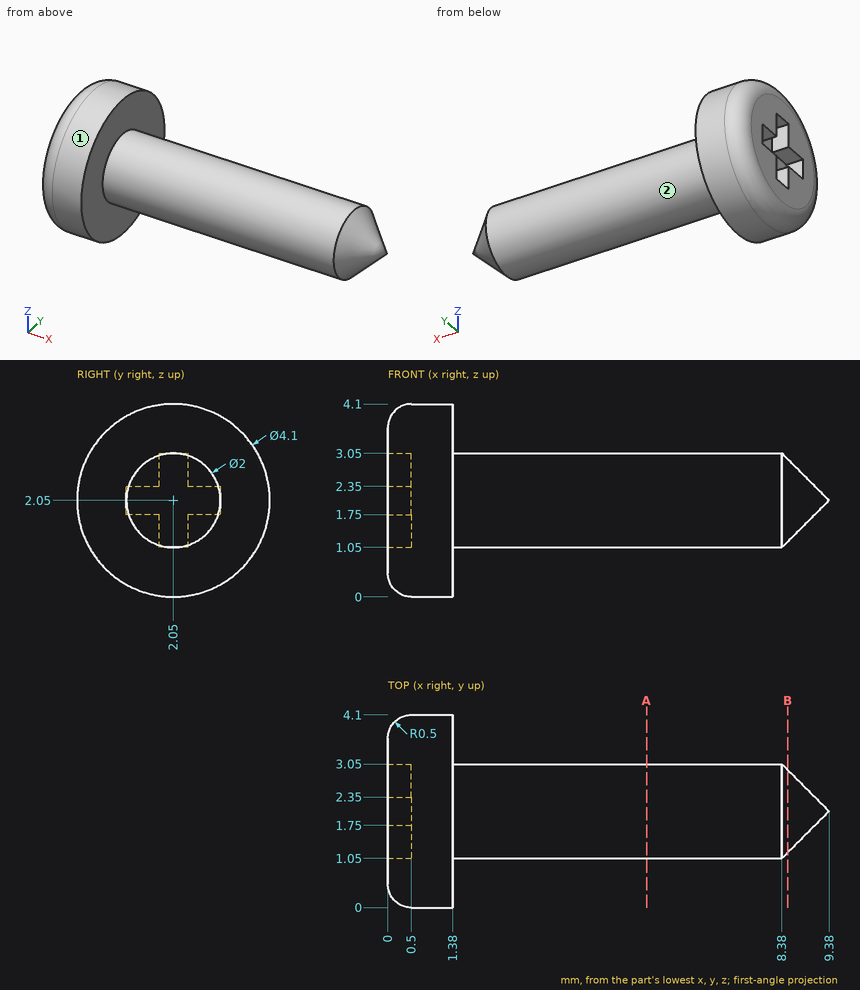
Input: dimensioned drawing with shaded views. Units: mm. Origin: part minimum x, y, z. A direction names the side the tool comes from. Give positions to 0.01 mm unless a question says otherwise; leave off trailing zeros. Write each loop counter-clockwise with the first axis right and the second up, starting at its lowest first coordinate (ties: lowest second). Pieces come first, ordered by that corner, then holes. Notation, with made-up numbers: (0.5, 41.5) - (12.5, 41.5) arc R22 cw to (12.5, 52.5) - close; hole circle Ø11 at (-38.5, 33.25). An arc over 180 degrees is marked (long way). One line per item, written item: value. Start each with the question number.
Q1. Material intervals for probe 1 along X at (y, z) = (1.4, 0.75); probe 2 along Y at (x, z) = (3, 1.2); probe 3 along Z at (x, y) = (3, 1.8), sorted ascending. Write a range as from..to.
Q2. Set-up query: the marked faces 1 and 2. Return all of +Z, -Z, +X, -X, +Y, -Y with unobstructed straight access to the full face (end or side cutting, diameter ignored); none if empty.
Q3. Section query A-A, the plane x = 5.5. Return the cut outline in (y, z).
Q4. Section query B-B, the plane x = 8.5. Return the cut outline in (y, z), then the cut area to 3 significant figures.
Q5. First-contact query: pin 1 Ø1 at (y, z) = (2.5, 0.5) entering from +X; pin 2 Ø1 at (x, z) = (6.5, 1.5) entering from +Y; pin 3 Ø1.5 at (x, z) = (4, 2) entering from -Y. Flat tips, straight axial feed; report the tip coordinate or a pass-through.
Answer:
1. probe 1: x = 0..1.38
1. probe 2: y = 1.52..2.58
1. probe 3: z = 1.08..3.02
2. face 1: +X, -X
2. face 2: +X
3. outline: circle Ø2 at (2.05, 2.05)
4. outline: circle Ø1.76 at (2.05, 2.05)
4. area: 2.43 mm2
5. pin 1: stops at x = 1.38
5. pin 2: stops at y = 3.05
5. pin 3: stops at y = 1.05
